Verification items for the finished model (mm, model axes). Face numbers are marked on the shaded views. Give positions to 0.01 mm unless a question says otherwise; leave off trailing zeros. Write each loop counter-clockwise with the first axis right and the second up, starting at its lowest first coordinate (ties: lowest second). Pieces come first, ordered by that corner, then holes. Notation, with made-up numbers: (68.5, 48) -> (90.5, 48) arc R10 ccw to (90.5, 67) -> close; hole circle Ø10 at (2, 70). An arc over 180 degrees is marked (long way). Answer as CSV lines item,"result". Start each with the question number.
1) Sectioned sample at A-A on x = 0. Record the cut outline in (y, z) (3 decimals), and give its area (4 significant figures).
2) Sectioned sample at B-B on z = 0. Record the cut outline in (x, y) (3 decimals).
3) Material ranges on L1, parallel to Z at x = 0, y = 8.25 (3 decimals); L2, parallel to X at y = 6, z = 0.25; L3, parallel to Y at x = -9.5, z = -3.5, recorded low to high.
4) Sectioned sample at C-C on y = 8.25. Record the cut outline in (x, z) (3 decimals), and give its area (3 significant figures).
5) Mould release check, pull along Z, two halves, no side actions. Record for the marked faces 1, 2 and 3: released by +Z, released by -Z, zero draft, split by the parting line, or undercut.
6) Gauge pin test, flat ends, axial feed: pin 1 Ø1.5 at (x, y) = (6, 8) entering from +Z; pin 2 Ø3 at (y, z) = (7.5, 2) entering from -X; pin 3 Ø3 at (y, z) = (4.5, 3) entering from -X; pin 4 Ø4 at (x, y) = (-1.5, 3) entering from +Z (3 decimals). Record the tip position at first contact, or that the pin passes through.
7) Sectioned sample at D-D on y = 1.25. Record the cut outline in (x, z) (3 decimals).
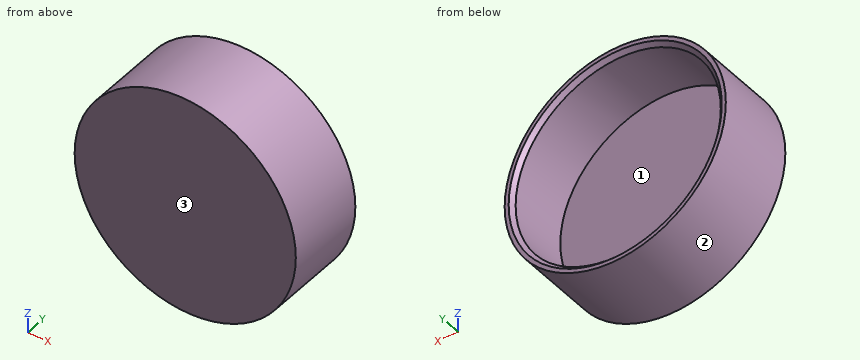
Autodesk Inventor part; units mm, degrees
ref_plane "YZ Plane" through (0, 0, 0) normal (1, 0, 0) x (0, 1, 0)
ref_plane "XZ Plane" through (0, 0, 0) normal (0, 1, 0) x (-1, 0, 0)
ref_plane "XY Plane" through (0, 0, 0) normal (0, 0, 1) x (1, 0, 0)
sketch "Sketch1" plane through (0, 0, 0) normal (0, 1, 0) x (-1, 0, 0)
  circle A0 centre (0, 0) radius 12.825
  circle A1 centre (0, 0) radius 13.825
  dimension "d0" = 25.65
  dimension "d1" = 27.65
extrude "Extrusion1" add sketch "Sketch1" along normal blind 10 contours A0 | A1
sketch "Sketch3" plane through (0, 10, 0) normal (0, 1, 0) x (1, 0, 0)
  circle A0 centre (0, 0) radius 12.825
  circle A1 centre (0, 0) radius 13.825
  dimension "d11" = 25.65
  dimension "d12" = 27.65
extrude "Extrusion3" cut sketch "Sketch3" against normal blind 8 contours A0
chamfer "Chamfer2" distance 0.5 angle 45 1 edges at (-12.825, 10, 0)
properties part number "TubeCap"
Ans:
1,outline,"(0, -13.825) -> (10, -13.825) -> (10, -13.325) -> (9.5, -12.825) -> (2, -12.825) -> (2, 12.825) -> (9.5, 12.825) -> (10, 13.325) -> (10, 13.825) -> (0, 13.825) -> close"
1,area,"71.05 mm²"
2,outline,"(-13.825, 0) -> (13.825, 0) -> (13.825, 10) -> (13.325, 10) -> (12.825, 9.5) -> (12.825, 2) -> (-12.825, 2) -> (-12.825, 9.5) -> (-13.325, 10) -> (-13.825, 10) -> close"
3,L1,"z = -13.825 to -12.825, 12.825 to 13.825"
3,L2,"x = -13.82 to -12.82, 12.82 to 13.82"
3,L3,"y = 0 to 2"
4,outline,"circle Ø27.65 at (0, 0); hole circle Ø25.65 at (0, 0)"
4,area,"83.7 mm²"
5,face 1,"undercut"
5,face 2,"split by the parting line"
5,face 3,"zero draft"
6,pin 1,"stops at z = 12.79"
6,pin 2,"stops at x = -13.82"
6,pin 3,"stops at x = -13.74"
6,pin 4,"stops at z = 13.825"
7,outline,"circle Ø27.65 at (0, 0)"
